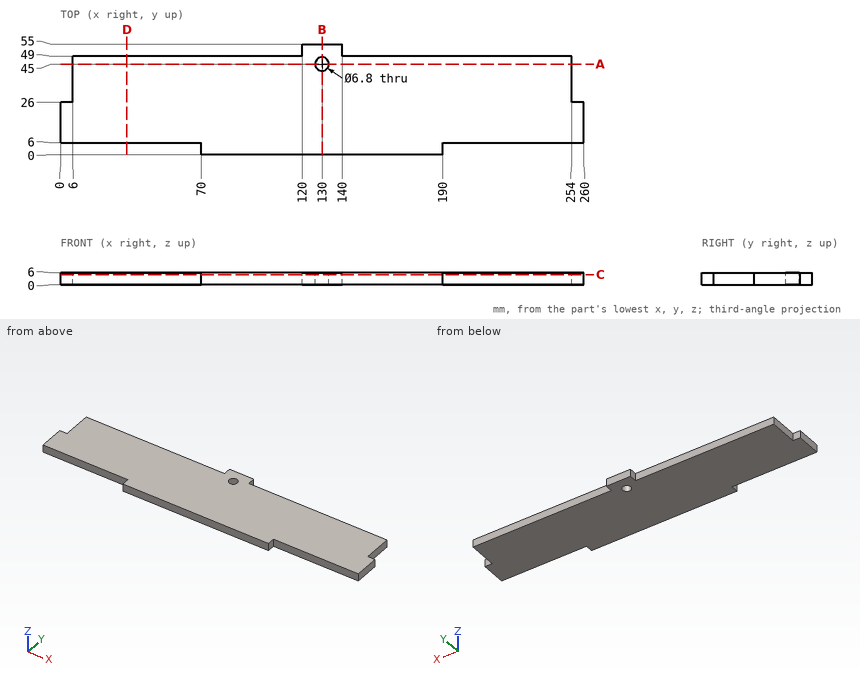
Geometry: see drawing. Coordinates: mm, zero at the bounding-box minimum. Coordinates: 2 decimals unless noted, no trailing zeros. Loops run counter-clockwise (first coordinate to the right, second up) from the corner with the lowest first, then second, coordinate; pieces in that order, holes last. Notation, with made-up numbers: M 22,76.5 L 31,76.5 A35 ccw 31,113.5 Z; hole C 74.25,-25.75 d2. An arc over 180 degrees is marked long. Answer in a Markdown table with one row per item.
Q1. Section D-D on x = 33. Return the cut outline in (y, z), plus the area to 3 significant figures.
Answers below:
| item | result |
|---|---|
| outline | M 6,0 L 49,0 L 49,6 L 6,6 Z |
| area | 258 mm^2 |
Q2. First-contact query: pin 1 (1.8 mm diameter, centred on y = 32, z = 2, fed in from +X); pin 2 (1.8 mm diameter, centred on y = 37, z = 4.5, fed in from -X); pin 3 (3 mm diameter, centred on x = 19.5, z = 3, fed in from -Y); pin 4 (6 mm diameter, centred on x = 130, y = 45, fed in from +Z). Flat tips, straight axial feed; report the tip coordinate or a pass-through.
Answers below:
| item | result |
|---|---|
| pin 1 | stops at x = 254 |
| pin 2 | stops at x = 6 |
| pin 3 | stops at y = 6 |
| pin 4 | passes through |
Q3. Section A-A on y = 45. Return the cut outline in (x, z).
Answers below:
| item | result |
|---|---|
| outline | M 6,0 L 126.6,0 L 126.6,6 L 6,6 Z; M 133.4,0 L 254,0 L 254,6 L 133.4,6 Z |
Q4. Section B-B on x = 130. Return the cut outline in (y, z).
Answers below:
| item | result |
|---|---|
| outline | M 0,0 L 41.6,0 L 41.6,6 L 0,6 Z; M 48.4,0 L 55,0 L 55,6 L 48.4,6 Z |
Q5. Ray query, probe 1 along Y at (x, z) = (130, 3.1); probe 2 along Y at (x, z) = (243, 2.5); probe 3 along X at (y, z) = (33, 4.2). Return the intervals inside material, ascending. Write a range as from..to.
Answers below:
| item | result |
|---|---|
| probe 1 | y = 0..41.6, 48.4..55 |
| probe 2 | y = 6..49 |
| probe 3 | x = 6..254 |
Q6. Section C-C on z = 5. Return the cut outline in (x, y), plus the area to 3 significant figures.
Answers below:
| item | result |
|---|---|
| outline | M 0,6 L 70,6 L 70,0 L 190,0 L 190,6 L 260,6 L 260,26 L 254,26 L 254,49 L 140,49 L 140,55 L 120,55 L 120,49 L 6,49 L 6,26 L 0,26 Z; hole C 130,45 d6.8 |
| area | 11,700 mm^2 |
